```python
from build123d import *

# Parameters (mm, degrees)
EXTRUDE_1_DEPTH          = 60
CUT_EXTRUDE_1_DEPTH      = 40
CUT_EXTRUDE_1_DEPTH_BACK = 29
SKETCH_4_R               = 15.5
SKETCH_5_W               = 5
SKETCH_5_H               = 30
CUT_EXTRUDE_2_DEPTH      = 83.900874001
SKETCH_7_W               = 60
SKETCH_7_H               = 85.424918669
EXTRUDE_2_DEPTH          = 17
CUT_EXTRUDE_START        = -34.454396
SKETCH_9_W               = 21
SKETCH_9_H               = 40.17
CUT_EXTRUDE_3_DEPTH      = 14
SKETCH_12_W              = 60
SKETCH_12_H              = 16.92976669
CUT_EXTRUDE_4_DEPTH      = 120.781279465
CUT_EXTRUDE_START_2      = -15
SKETCH_14_W              = 60
SKETCH_14_H              = 56
CUT_EXTRUDE_8_DEPTH      = 10


with BuildPart() as part:
    # 스케치3 → 보스-돌출1 (new body)
    with BuildSketch(Plane(origin=(0, 0, 0), x_dir=(0, 0, -1), z_dir=(1, 0, 0))):
        Polygon((-25, -51.454396413), (25, -51.454396413), (15, 4.545603587), (-15, 4.545603587), align=None)
    extrude(amount=EXTRUDE_1_DEPTH)

    # 스케치4 → 컷-돌출1 (cut, two sides: drawn at the far end of the back side and taken through both)
    with BuildSketch(Plane.XY.offset(-CUT_EXTRUDE_1_DEPTH_BACK)):
        with Locations(Location((30, -14.954396413, 0), (0, 0, 90))):
            Circle(SKETCH_4_R)
    extrude(amount=CUT_EXTRUDE_1_DEPTH + CUT_EXTRUDE_1_DEPTH_BACK, mode=Mode.SUBTRACT)

    # 스케치5 → 컷-돌출2 (cut, through all)
    with BuildSketch(Plane(origin=(0, 0, 0), x_dir=(0, 0, -1), z_dir=(1, 0, 0))):
        with Locations((0, -51.454396413)):
            Rectangle(SKETCH_5_W, SKETCH_5_H)
    extrude(amount=CUT_EXTRUDE_2_DEPTH, mode=Mode.SUBTRACT)

    # 스케치7 → 보스-돌출2 (add)
    with BuildSketch(Plane(origin=(0, -51.454396413, 0), x_dir=(-1, 0, 0), z_dir=(0, -1, 0))):
        with Locations((-30, -47.287540666)):
            Rectangle(SKETCH_7_W, SKETCH_7_H)
    extrude(amount=-EXTRUDE_2_DEPTH)

    # 스케치9 → 컷-돌출3 (cut)
    with BuildSketch(Plane(origin=(0, 0, 0), x_dir=(1, 0, 0), z_dir=(0, 1, 0)).offset(CUT_EXTRUDE_START)):
        with Locations((30, -42.049285714)):
            Rectangle(SKETCH_9_W, SKETCH_9_H)
    extrude(amount=-CUT_EXTRUDE_3_DEPTH, mode=Mode.SUBTRACT)

    # 스케치12 → 컷-돌출4 (cut, through all)
    with BuildSketch(Plane(origin=(0, 0, 0), x_dir=(1, 0, 0), z_dir=(0, 1, 0))):
        with Locations((30, -81.535116655)):
            Rectangle(SKETCH_12_W, SKETCH_12_H)
    extrude(amount=-CUT_EXTRUDE_4_DEPTH, mode=Mode.SUBTRACT)

    # 스케치14 → 컷-돌출8 (cut)
    with BuildSketch(Plane.XY.offset(CUT_EXTRUDE_START_2)):
        with Locations((30, -23.454396413)):
            Rectangle(SKETCH_14_W, SKETCH_14_H)
    extrude(amount=-CUT_EXTRUDE_8_DEPTH, mode=Mode.SUBTRACT)


solid = part.part
```
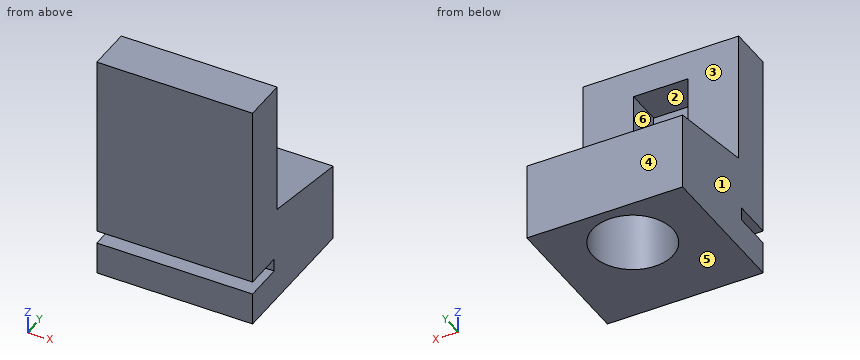
The listing builds one solid part. Answer for the finished solid, in the listing's coordinates (mm). Face numbers are marked on the shaded views. A direction names the side the tool comes from. Round coordinates to 2 decimals unless told otherwise and drop trailing zeros. Write each loop counter-clockwise with the first axis right and the second up, starting at its lowest first coordinate (ties: lowest second). Pieces come first, ordered by that corner, then holes. Notation, with made-up numbers: (-4.5, 15) -> (10.5, 15) arc R22 cw to (10.5, 49) -> close; hole circle Ø5 at (71, -26.5). An arc over 180 degrees is marked (long way). Answer as a JSON object with one key per item and string values. Group by question number.
Q1. Section D-D (y = -3.5) is taken. Write down the section's boundary in (x, z), plus the area to 3 significant figures.
Q2. Determine the mould class of the marked faces 4, 5 and 6 for opening direction Z: pulls with the +Z half, pulls with the -Z half, needs draft (parallel to the pull), parting line crosses it, or undercut.
Q3. Section C-C (x = 30) is taken. Write down the section's boundary in (y, z), plus the area to 3 significant figures.
Q4. Section A-A (y = -40.5) is taken. Write down the section's boundary in (x, z).
Q5. Straight lines are drawn through the part: line 1 along Z through (x, y) = (25, -37); line 2 along Z through (x, y) = (49, -47); line 3 along X through (y, z) = (-48, 34.5). For each, find the intervals that lie inside material, in ascending order.
Q6. Section B-B (x = 6) is taken. Write down the section's boundary in (y, z).
Q7. Which of the six approach directions +Z, -Z, +X, -X, +Y, -Y give full straight-line access (tool end or side, diameter ignored) to the marked faces 1, 2 and 3?
Q8. Each of these flat-tipped pins is pushed along its axis until it touches: pin 1 Ø6 at (x, z) = (13.5, 36) entering from +Y; pin 2 Ø3 at (x, z) = (27, 59.5) entering from +Y; pin 3 Ø6 at (x, y) = (8.5, -14.5) entering from +Z. Where does it stop, or does it pass through?
Check values:
{
 "1": {"outline": "(0, -15) -> (19.56, -15) -> (19.56, 16.44) -> (0, 16.44) -> close; (40.44, -15) -> (60, -15) -> (60, 16.44) -> (40.44, 16.44) -> close", "area": "1,230 mm^2"},
 "2": {"face 4": "needs draft", "face 5": "pulls with the -Z half", "face 6": "undercut"},
 "3": {"outline": "(-51.45, -15) -> (-30.45, -15) -> (-30.45, 21.25) -> (-34.45, 21.96) -> (-48.45, 21.96) -> (-48.45, 62.13) -> (-34.45, 62.13) -> (-34.45, 73.07) -> (-51.45, 73.07) -> (-51.45, 2.5) -> (-36.45, 2.5) -> (-36.45, -2.5) -> (-51.45, -2.5) -> close; (0.55, -15) -> (4.55, -15) -> (4.55, 15) -> (0.55, 15.71) -> close", "area": "1,130 mm^2"},
 "4": {"outline": "(0, -15) -> (60, -15) -> (60, -2.5) -> (0, -2.5) -> close; (0, 2.5) -> (60, 2.5) -> (60, 73.07) -> (0, 73.07) -> close; hole (19.5, 21.96) -> (40.5, 21.96) -> (40.5, 62.13) -> (19.5, 62.13) -> close"},
 "5": {"line 1": "-15 to -2.5, 2.5 to 21.96, 62.13 to 73.07", "line 2": "-15 to -2.5, 2.5 to 73.07", "line 3": "0 to 19.5, 40.5 to 60"},
 "6": {"outline": "(-51.45, -15) -> (4.55, -15) -> (4.55, 15) -> (-34.45, 21.96) -> (-34.45, 73.07) -> (-51.45, 73.07) -> (-51.45, 2.5) -> (-36.45, 2.5) -> (-36.45, -2.5) -> (-51.45, -2.5) -> close"},
 "7": {"face 1": "+Z, -Z, -X, +Y, -Y", "face 2": "+Y", "face 3": "+Z, +X, -X, +Y"},
 "8": {"pin 1": "y = -34.45", "pin 2": "y = -48.45", "pin 3": "z = 18.94"}
}
